```python
from build123d import *

# Parameters (mm, degrees)
F2_W     = 150
F2_H     = 10
F3_DEPTH = 50
F5_DEPTH = 203
F6_W     = 66.240772
F6_H     = 165
F7_DEPTH = 1
F8_R     = 5


with BuildPart() as f1:
    # F0 (on Right) → F1 (revolve)
    with BuildSketch(Plane.YZ):
        with BuildLine():
            ThreePointArc((-170.446234, 17.055093), (-177.448849, 9.774337), (-180, 0))
            Line((-180, 0), (180, 0))
            ThreePointArc((180, 0), (177.448849, 9.774337), (170.446234, 17.055093))
            ThreePointArc((170.446234, 17.055093), (0, 65.105742), (-170.446234, 17.055093))
        make_face()
    revolve(axis=Axis((0, 0, 0), (0, 1, 0)))

    # F2 (on Right) → F3 (cut, symmetric)
    with BuildSketch(Plane.YZ):
        with Locations((0, -65)):
            Rectangle(F2_W, F2_H)
        Polygon((75, 70), (-75, 70), (-75, 60), (0, 60), (75, 60), align=None)
    extrude(amount=F3_DEPTH, both=True, mode=Mode.SUBTRACT)

    # F4 (on Front) → F5 (cut, symmetric)
    with BuildSketch(Plane.XZ):
        Polygon((68.942911, -68.942911), (-68.942911, 68.942911), (-68.942911, -68.942911), align=None)
    extrude(amount=F5_DEPTH, both=True, mode=Mode.SUBTRACT)

    # F6 (on face) → F7 (cut)
    with BuildSketch(Plane(origin=(0, 0, 0), x_dir=(0.707107, 0, -0.707107), z_dir=(-0.707107, 0, -0.707107))):
        Rectangle(F6_W, F6_H)
    extrude(amount=-F7_DEPTH, mode=Mode.SUBTRACT)

    # F8
    f8_edges = [f1.edges().sort_by_distance(p)[0] for p in [
        (0, -57.5, 60),
    ]]
    fillet(f8_edges, radius=F8_R)


solid = f1.part
```
For this review, take the finished solid that the model builds, in its own axes (mm). Give positions to 0.01 mm unless a question says otherwise; leave off trailing zeros.
1) Wall thickness on line 1 (Z direction, x = -21, y = -73.5); line 2 (Y direction, x = -7.5, z = 13); line 3 (X direction, y = -72, z = 17): over which ranges is each line inside the solid? List them lowest first.
2) Insertion check: pin 1 (1 mm diameter, centred on x = 18, z = 17, fed in from +Y); pin 2 (1 mm diameter, centred on x = -11, y = 113, fed in from +Z); pin 3 (6 mm diameter, centred on x = 22.5, y = -93.5, fed in from +Z). Each pin has a flat end and moves straight along its axis. Give the tip position at first contact, or say it passes through.
3) The part is to be moulded in two halves that separate along Y. For faces 1 (the face through (0, 82.5, 1)), 2 (the face through (-30, -3, 30)), say which applies: released by +Y, released by -Y, zero draft, split by the parting line, or undercut.
Derived:
1. line 1: z = 22.41 to 52.69
1. line 2: y = -173.22 to 173.22
1. line 3: x = -15.59 to 54.47
2. pin 1: stops at y = 158.08
2. pin 2: stops at z = 43.78
2. pin 3: stops at z = 47.91
3. face 1: undercut
3. face 2: zero draft
